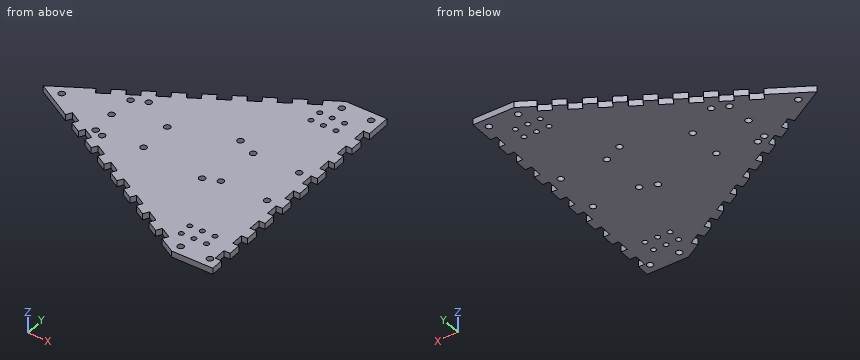
```python
from build123d import *

# Parameters (mm, degrees)
SKETCH1_R               = 2
BOSS_EXTRUDE1_DEPTH     = 5
SKETCH2_R               = 2.5
CUT_EXTRUDE1_DEPTH      = 1
CUT_EXTRUDE1_DEPTH_BACK = 6
SKETCH3_R               = 2.5
SKETCH3_W               = 5
SKETCH3_H               = 10
CUT_EXTRUDE5_DEPTH      = 1
CUT_EXTRUDE5_DEPTH_BACK = 6


with BuildPart() as part:
    # Sketch1 → Boss-Extrude1 (new body)
    with BuildSketch(Plane.XY):
        Polygon((2.5, 0), (-30.5, 0), (-203.705080757, -100), (-30.5, -200), (2.5, -200), align=None)
        with Locations((-17.5, -20)):
            Circle(SKETCH1_R, mode=Mode.SUBTRACT)
        with Locations((-27.5, -20)):
            Circle(SKETCH1_R, mode=Mode.SUBTRACT)
        with Locations((-37.5, -20)):
            Circle(SKETCH1_R, mode=Mode.SUBTRACT)
        with Locations((-27.5, -30)):
            Circle(SKETCH1_R, mode=Mode.SUBTRACT)
        with Locations((-37.5, -30)):
            Circle(SKETCH1_R, mode=Mode.SUBTRACT)
        with Locations((-17.5, -30)):
            Circle(SKETCH1_R, mode=Mode.SUBTRACT)
        with Locations((-36.32829598, -180.575203576)):
            Circle(SKETCH1_R, mode=Mode.SUBTRACT)
        with Locations((-26.329360823, -180.429272995)):
            Circle(SKETCH1_R, mode=Mode.SUBTRACT)
        with Locations((-26.475291404, -170.430337839)):
            Circle(SKETCH1_R, mode=Mode.SUBTRACT)
        with Locations((-16.476356247, -170.284407258)):
            Circle(SKETCH1_R, mode=Mode.SUBTRACT)
        with Locations((-16.330425667, -180.283342414)):
            Circle(SKETCH1_R, mode=Mode.SUBTRACT)
        with Locations((-36.474226561, -170.576268419)):
            Circle(SKETCH1_R, mode=Mode.SUBTRACT)
    extrude(amount=BOSS_EXTRUDE1_DEPTH)

    # Sketch2 → Cut-Extrude1 (cut, two sides)
    with BuildSketch(Plane.XY.offset(5)) as cut_extrude1_sk:
        with Locations((-188.705080757, -100)):
            Circle(SKETCH2_R)
        with Locations((-5, -192.5)):
            Circle(SKETCH2_R)
        with Locations((-10.85, -118.605720398)):
            Circle(SKETCH2_R)
        with Locations((-47.85, -118.605720398)):
            Circle(SKETCH2_R)
        with Locations((-5, -7.5)):
            Circle(SKETCH2_R)
        with Locations((-47.85, -81.605720398)):
            Circle(SKETCH2_R)
        with Locations((-28.490381057, -192.5)):
            Circle(SKETCH2_R)
        with Locations((-10.85, -81.605720398)):
            Circle(SKETCH2_R)
        with Locations((-28.490381057, -7.5)):
            Circle(SKETCH2_R)
    extrude(amount=CUT_EXTRUDE1_DEPTH, mode=Mode.SUBTRACT)
    extrude(cut_extrude1_sk.sketch, amount=-CUT_EXTRUDE1_DEPTH_BACK, mode=Mode.SUBTRACT)

    # Sketch3 → Cut-Extrude5 (cut, two sides)
    with BuildSketch(Plane.XY.offset(5)) as cut_extrude5_sk:
        with Locations((-136.253175473, -75)):
            Circle(SKETCH3_R)
        with Locations((-62.653175473, -75)):
            Circle(SKETCH3_R)
        with Locations((-140.495575744, -122.5)):
            Circle(SKETCH3_R)
        with Locations((-59.775575744, -123.169872981)):
            Circle(SKETCH3_R)
        with Locations((-110.745575744, -117.5)):
            Circle(SKETCH3_R)
        with Locations((-110.745575744, -90.25)):
            Circle(SKETCH3_R)
        with Locations((-148.705080757, -100)):
            Circle(SKETCH3_R)
        with Locations((-147.413429511, -80)):
            Circle(SKETCH3_R)
        with Locations((-147.413429511, -120)):
            Circle(SKETCH3_R)
        Polygon((-121.432667397, -52.5), (-112.77241336, -47.5), (-110.27241336, -51.830127019), (-118.932667397, -56.830127019), align=None)
        Polygon((-101.612159322, -46.830127019), (-104.112159322, -42.5), (-95.451905284, -37.5), (-92.951905284, -41.830127019), align=None)
        Polygon((-84.291651246, -36.830127019), (-86.791651246, -32.5), (-78.131397208, -27.5), (-75.631397208, -31.830127019), align=None)
        Polygon((-66.97114317, -26.830127019), (-69.47114317, -22.5), (-60.810889132, -17.5), (-58.310889132, -21.830127019), align=None)
        Polygon((-49.650635095, -16.830127019), (-52.150635095, -12.5), (-43.490381057, -7.5), (-40.990381057, -11.830127019), align=None)
        Polygon((-136.253175473, -66.830127019), (-138.753175473, -62.5), (-130.092921435, -57.5), (-127.592921435, -61.830127019), align=None)
        Polygon((-153.573683549, -76.830127019), (-156.073683549, -72.5), (-147.413429511, -67.5), (-144.913429511, -71.830127019), align=None)
        Polygon((-170.894191624, -86.830127019), (-173.394191624, -82.5), (-164.733937587, -77.5), (-162.233937587, -81.830127019), align=None)
        Polygon((-112.77241336, -152.5), (-110.27241336, -148.169872981), (-118.932667397, -143.169872981), (-121.432667397, -147.5), align=None)
        Polygon((-173.394191624, -117.5), (-164.733937587, -122.5), (-162.233937587, -118.169872981), (-170.894191624, -113.169872981), align=None)
        Polygon((-156.073683549, -127.5), (-147.413429511, -132.5), (-144.913429511, -128.169872981), (-153.573683549, -123.169872981), align=None)
        Polygon((-138.753175473, -137.5), (-130.092921435, -142.5), (-127.592921435, -138.169872981), (-136.253175473, -133.169872981), align=None)
        Polygon((-52.150635095, -187.5), (-43.490381057, -192.5), (-40.990381057, -188.169872981), (-49.650635095, -183.169872981), align=None)
        Polygon((-69.47114317, -177.5), (-60.810889132, -182.5), (-58.310889132, -178.169872981), (-66.97114317, -173.169872981), align=None)
        Polygon((-86.791651246, -167.5), (-78.131397208, -172.5), (-75.631397208, -168.169872981), (-84.291651246, -163.169872981), align=None)
        Polygon((-104.112159322, -157.5), (-95.451905284, -162.5), (-92.951905284, -158.169872981), (-101.612159322, -153.169872981), align=None)
        with Locations((0, -85)):
            Rectangle(SKETCH3_W, SKETCH3_H)
        with Locations((0, -105)):
            Rectangle(SKETCH3_W, SKETCH3_H)
        with Locations((0, -65)):
            Rectangle(SKETCH3_W, SKETCH3_H)
        with Locations((0, -45)):
            Rectangle(SKETCH3_W, SKETCH3_H)
        with Locations((0, -25)):
            Rectangle(SKETCH3_W, SKETCH3_H)
        with Locations((0, -125)):
            Rectangle(SKETCH3_W, SKETCH3_H)
        with Locations((0, -145)):
            Rectangle(SKETCH3_W, SKETCH3_H)
        with Locations((0, -165)):
            Rectangle(SKETCH3_W, SKETCH3_H)
        with Locations((0, -185)):
            Rectangle(SKETCH3_W, SKETCH3_H)
    extrude(amount=CUT_EXTRUDE5_DEPTH, mode=Mode.SUBTRACT)
    extrude(cut_extrude5_sk.sketch, amount=-CUT_EXTRUDE5_DEPTH_BACK, mode=Mode.SUBTRACT)


solid = part.part
```
Part model, mm, in its own coordinate system. Round coordinates to 2 decimals unless told otherwise and drop trailing zeros. Return JSON: item names as keys, results as strings. Group by question number.
Q1. Probe L1, parallel to X at y = -192.5, z = 1.6; L2, parallel to Y at x = -10.85, z = 3.65; L3, parallel to Y at x = -5, z = 1.4. List the from-to ranges inside material, lowest first. Write a range as [from, to].
Q2. Saw through at A-A on z = 3.7. State how many separate pieces and enclosed holes the cut face has, plus the area to 3 significant figures.
Q3. Pin check, flat tips, straight feed: pin 1 (2.5 mm diameter, centred on x = 0, z = 2, fed in from +Y); pin 2 (1 mm diameter, centred on x = -90, z = 1.5, fed in from -Y); pin 3 (1.5 mm diameter, centred on x = -108, z = 4, fed in from -Y); pin 4 (3 mm diameter, centred on y = -64.5, z = 2.5, fed in from +X). Stop position of each tip, or through.
Answer:
{
 "1": {"L1": "[-43.49, -30.99], [-25.99, -7.5], [-2.5, 2.5]", "L2": "[-200, -121.11], [-116.11, -84.11], [-79.11, 0]", "L3": "[-200, -195], [-190, -10], [-5, 0]"},
 "2": {"separate pieces": "1", "enclosed holes": "30", "area": "22,200 mm2"},
 "3": {"pin 1": "y = 0", "pin 2": "y = -165.94", "pin 3": "y = -155.69", "pin 4": "x = -2.5"}
}
